```python
from build123d import *

# Parameters (mm, degrees)
PAD_DEPTH = 3
FILLET_R  = 2


with BuildPart() as part:
    # Sketch → Pad (new body)
    with BuildSketch(Plane.XY):
        with BuildLine():
            Line((-15.560135, 12.975312), (-25.739783, 6.963025))
            ThreePointArc((-25.739783, 6.963025), (-28.010173, 2.501983), (-24.932128, -1.44532))
            Line((-24.932128, -1.44532), (-17.320507, -13.22905))
            Line((-17.320507, -13.22905), (-14.701975, 2.263941))
            Line((-14.701975, 2.263941), (-6.95548, 1.718414))
            Line((-6.95548, 1.718414), (-7.991983, -3.082232))
            Line((-7.991983, -3.082232), (2.318496, -7.719219))
            Line((2.318496, -7.719219), (13.665469, 2.536705))
            Line((13.665469, 2.536705), (6.846373, 4.227841))
            Line((6.846373, 4.227841), (19.792001, 11.370732))
            Line((19.792001, 11.370732), (7.520889, 15.262908))
            ThreePointArc((7.520889, 15.262908), (-4.255017, 16.494155), (-15.560135, 12.975312))
        make_face()
    extrude(amount=PAD_DEPTH)

    # Fillet
    fillet_edges = [part.edges().sort_by_distance(p)[0] for p in [
        (-14.701975, 2.263941, 1.5),
        (-6.95548, 1.718414, 1.5),
        (-7.991983, -3.082232, 1.5),
        (6.846373, 4.227841, 1.5),
    ]]
    fillet(fillet_edges, radius=FILLET_R)


solid = part.part
```
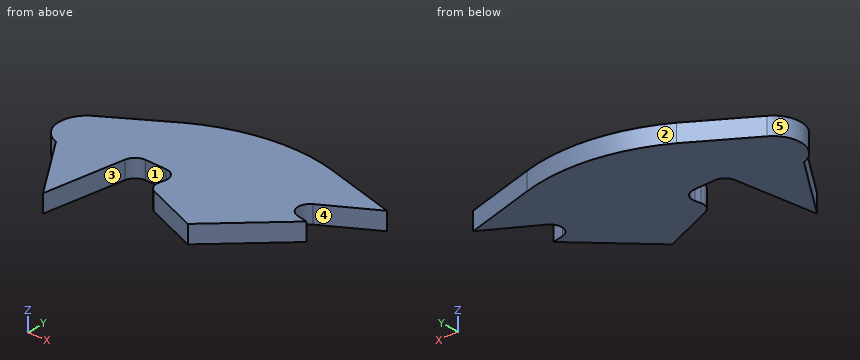
Source: CAD feature listing. Evaluate the final solid. Frame: model axes, mm. Face numbers are marked on the shaded views. A direction names the side the tool comes from. Round coordinates to 2 decimals unless told otherwise and drop trailing zeros. Loops run counter-clockwise (first coordinate to the right, second up) from the corner with the lowest first, then second, coordinate; pieces in that order, holes last. Notation, with made-up numbers: M 20.5,-21.75 L 79.5,-21.75 A14 cw 79.5,2.25 Z; hole C 66.25,6 d3. An arc over 180 degrees is marked long. Use a Markdown table: item, result. Add a question column.
1. Cut plane B-B, the plane z = 1.1. Output: boundary loops of the cut face in (x, y).
2. Cut plane C-C, the plane y = -5. Output: boundary loops of the cut face in (x, z), and give its area (3 significant figures).
3. Set-up query: the marked faces 1 and 2. Return all of +Z, -Z, +X, -X, +Y, -Y with unobstructed straight access to the full face (end or side cutting, diameter ignored); none if empty.
4. Contact query for a flat-ended pin moving along its axis: pin 1 (1 mm diameter, centred on x = 1, z = 1, fed in from +Y). Output: stop coordinate, or through.
5. Cut plane D-D, the plane x = -22. Output: boundary loops of the cut face in (y, z).
6. Ray query, line 1 along X through (y, z) = (1.5, 1.35); line 2 along X through (y, z) = (3.25, 1); line 3 along X through (y, z) = (8, 0.8). Return the intervals inside material, ascending. Write a range as [from, to].
7. Pull-direction query (Y, two-part tool) for the marked faces 3, 4 and 5; classes: +Y half, -Y half, draft (parallel to the pull), parting line (faces both ways), or undercut.
8. Cut plane A-A, the plane y = -2. Output: boundary loops of the cut face in (x, z), and give its area (3 significant figures).
Solution:
| question | item | result |
|---|---|---|
| 1 | outline | M -25.74,6.96 A4.66 ccw -24.93,-1.45 L -17.32,-13.23 L -15,0.47 A2 cw -12.89,2.14 L -9.26,1.88 A2 cw -7.44,-0.54 L -7.65,-1.5 A2 ccw -6.52,-3.75 L 2.32,-7.72 L 13.67,2.54 L 11.8,3 A2 cw 11.31,6.69 L 19.79,11.37 L 7.52,15.26 A29.37 ccw -15.56,12.98 Z |
| 2 | outline | M -22.64,0 L -15.93,0 L -15.93,3 L -22.64,3 Z; M -3.73,0 L 5.33,0 L 5.33,3 L -3.73,3 Z |
| 2 | area | 47.3 mm2 |
| 3 | face 1 | +Z, -Z, -Y |
| 3 | face 2 | +Z, -Z, +Y |
| 4 | pin 1 | stops at y = 16.58 |
| 5 | outline | M -5.98,0 L 9.17,0 L 9.17,3 L -5.98,3 Z |
| 6 | line 1 | x = [-27.8, -14.5], [-8.22, 12.52] |
| 6 | line 2 | x = [-28.02, 11.21] |
| 6 | line 3 | x = [-23.98, 13.68] |
| 7 | face 3 | -Y half |
| 7 | face 4 | undercut |
| 7 | face 5 | parting line |
| 8 | outline | M -24.57,0 L -15.42,0 L -15.42,3 L -24.57,3 Z; M -7.69,0 L 8.65,0 L 8.65,3 L -7.69,3 Z |
| 8 | area | 76.5 mm2 |
